Could you check a few things on this model? Use its own coordinates, in mm. A direction names the side the tool comes from. Coordinates: 2 decimals unless noted, no trailing zeros. Write each loop counter-clockwise with the first axis right and the second up, starting at its lowest first coordinate (ties: lowest second). Pieces come first, ordered by that corner, then holes. Notation, with made-up numbers: M -16,64 L 19,64 A21 cw 19,87 Z; hole C 37.5,-13 d11. An arc over 180 degrees is marked long. Write item = value, one per line.
```python
from build123d import *

# Parameters (mm, degrees)
SKETCH1_W                                            = 45
SKETCH1_H                                            = 48
BOSS_EXTRUDE1_DEPTH                                  = 6
SKETCH2_W                                            = 45
SKETCH2_H                                            = 15
BOSS_EXTRUDE2_DEPTH                                  = 10
CBORE_FOR_M3_HEXAGON_SOCKET_HEAD_CAP_SCR_D           = 3.4
CBORE_FOR_M3_HEXAGON_SOCKET_HEAD_CAP_SCR_DEPTH       = 15
CBORE_FOR_M3_HEXAGON_SOCKET_HEAD_CAP_SCR_CBORE_D     = 6
CBORE_FOR_M3_HEXAGON_SOCKET_HEAD_CAP_SCR_CBORE_DEPTH = 3.4
CBORE_FOR_M3_HEXAGON_SOCKET_HEAD_CAP_SCR_TIP         = 1.021463052
SKETCH6_W                                            = 5
SKETCH6_H                                            = 38
BOSS_EXTRUDE3_DEPTH                                  = 9
FILLET1_R                                            = 2
CBORE_FOR_M3_HEXAGON_SOCKET_HEAD_CAP_2_D             = 3.4
CBORE_FOR_M3_HEXAGON_SOCKET_HEAD_CAP_2_CBORE_D       = 6
CBORE_FOR_M3_HEXAGON_SOCKET_HEAD_CAP_2_CBORE_DEPTH   = 3.4
CHAMFER3_SIZE                                        = 3
CUT_EXTRUDE1_DEPTH                                   = 54.16013544
CUT_EXTRUDE1_DEPTH_BACK                              = 54.16013544
M3_TAPPED_HOLE1_D                                    = 2.5
M3_TAPPED_HOLE1_DEPTH                                = 4
M3_TAPPED_HOLE1_TIP                                  = 0.751075774


with BuildPart() as part:
    # Sketch1 → Boss-Extrude1 (new body)
    with BuildSketch(Plane.XY):
        Rectangle(SKETCH1_W, SKETCH1_H)
    extrude(amount=BOSS_EXTRUDE1_DEPTH)

    # Sketch2 → Boss-Extrude2 (add)
    with BuildSketch(Plane.XZ.offset(24)):
        with Locations((0, 7.5)):
            Rectangle(SKETCH2_W, SKETCH2_H)
    extrude(amount=-BOSS_EXTRUDE2_DEPTH)

    # CBORE for M3 Hexagon socket head cap scr
    with Locations(Plane(origin=(0, -14, 0), x_dir=(1, 0, 0), z_dir=(0, 1, 0))):
        with Locations((-11.5, -11.36), (11.5, -11.36)):
            CounterBoreHole(CBORE_FOR_M3_HEXAGON_SOCKET_HEAD_CAP_SCR_D / 2, CBORE_FOR_M3_HEXAGON_SOCKET_HEAD_CAP_SCR_CBORE_D / 2, CBORE_FOR_M3_HEXAGON_SOCKET_HEAD_CAP_SCR_CBORE_DEPTH, depth=CBORE_FOR_M3_HEXAGON_SOCKET_HEAD_CAP_SCR_DEPTH)
            with Locations((0, 0, -(CBORE_FOR_M3_HEXAGON_SOCKET_HEAD_CAP_SCR_DEPTH + CBORE_FOR_M3_HEXAGON_SOCKET_HEAD_CAP_SCR_TIP / 2))):  # 118° drill point
                Cone(0, CBORE_FOR_M3_HEXAGON_SOCKET_HEAD_CAP_SCR_D / 2, CBORE_FOR_M3_HEXAGON_SOCKET_HEAD_CAP_SCR_TIP, mode=Mode.SUBTRACT)

    # Sketch6 → Boss-Extrude3 (add)
    with BuildSketch(Plane.XY.offset(6)):
        with Locations((-20, 5)):
            Rectangle(SKETCH6_W, SKETCH6_H)
    extrude(amount=BOSS_EXTRUDE3_DEPTH)

    # Fillet1
    fillet1_edges = [part.edges().sort_by_distance(p)[0] for p in [
        (-17.5, -14, 10.5),
    ]]
    fillet(fillet1_edges, radius=FILLET1_R)

    # CBORE for M3 Hexagon socket head cap 2 (through all)
    with Locations(Plane.XY.offset(6)):
        with Locations((0, 19), (0, 4)):
            CounterBoreHole(CBORE_FOR_M3_HEXAGON_SOCKET_HEAD_CAP_2_D / 2, CBORE_FOR_M3_HEXAGON_SOCKET_HEAD_CAP_2_CBORE_D / 2, CBORE_FOR_M3_HEXAGON_SOCKET_HEAD_CAP_2_CBORE_DEPTH)

    # Chamfer3
    chamfer3_edges = [part.edges().sort_by_distance(p)[0] for p in [
        (22.5, -24, 7.5),
        (-22.5, -24, 7.5),
    ]]
    chamfer(chamfer3_edges, length=CHAMFER3_SIZE)

    # Sketch9 → Cut-Extrude1 (cut, two sides: drawn at the far end of the back side and taken through both)
    with BuildSketch(Plane(origin=(22.5, 0, 0), x_dir=(0, 0, -1), z_dir=(1, 0, 0)).offset(-CUT_EXTRUDE1_DEPTH_BACK)):
        Polygon((74.04249055, 101.04249055), (-3, 24), (-15, 12), (-92.04249055, -65.04249055), (-246.12747165, 89.04249055), (-80.04249055, 255.12747165), align=None)
    extrude(amount=CUT_EXTRUDE1_DEPTH + CUT_EXTRUDE1_DEPTH_BACK, mode=Mode.SUBTRACT)

    # M3 Tapped Hole1
    with Locations(Plane.XY.offset(6)):
        with Locations((-12.5, 16), (17.5, 16), (-12.5, -9), (17.5, -9)):
            Hole(M3_TAPPED_HOLE1_D / 2, depth=M3_TAPPED_HOLE1_DEPTH)
            with Locations((0, 0, -(M3_TAPPED_HOLE1_DEPTH + M3_TAPPED_HOLE1_TIP / 2))):  # 118° drill point
                Cone(0, M3_TAPPED_HOLE1_D / 2, M3_TAPPED_HOLE1_TIP, mode=Mode.SUBTRACT)


solid = part.part
```
Item 1: If we mould it in two halves opening along Z, with no side actions, what happens to faces 1 (the face through (0, 0, 0)), 2 (the face through (10.586, -20.746, 9.927)), 3 (the face through (-12.3, -9.08, 1.38)), 4 (the face through (-12.414, -20.746, 9.927))? For each: pulls with the +Z half, pulls with the -Z half, needs draft (parallel to the pull), parting line crosses it, or undercut.
Numbers:
face_1 = pulls with the -Z half
face_2 = undercut
face_3 = pulls with the +Z half
face_4 = undercut
Item 2: Imagine slicing it at C-C (x = 0). Write out the boundary of the cut face in (y, z), and give its area (3 significant figures).
Numbers:
outline = M -24,0 L 2.3,0 L 2.3,2.6 L 1,2.6 L 1,6 L -14,6 L -14,15 L -24,15 Z; M 5.7,0 L 17.3,0 L 17.3,2.6 L 16,2.6 L 16,6 L 7,6 L 7,2.6 L 5.7,2.6 Z; M 20.7,0 L 24,0 L 24,3 L 22,5 L 22,2.6 L 20.7,2.6 Z
area = 316 mm²
Item 3: Imagine slicing it at A-A (x = 11.5). Write out the boundary of the cut face in (y, z), and give its area (3 significant figures).
Numbers:
outline = M -24,0 L 24,0 L 24,3 L 21,6 L -14,6 L -14,8.36 L -17.4,8.36 L -17.4,9.66 L -24,9.66 Z; M -24,13.06 L -17.4,13.06 L -17.4,14.36 L -14,14.36 L -14,15 L -24,15 Z
area = 331 mm²
Item 4: Imagine slicing it at B-B (z = 11.36). Write out the boundary of the cut face in (x, y).
Numbers:
outline = M -22.5,-21 L -19.5,-24 L -13.2,-24 L -13.2,-17.4 L -14.5,-17.4 L -14.5,-14 L -15.5,-14 A2 cw -17.5,-12 L -17.5,15.64 L -22.5,15.64 Z; M -9.8,-24 L 9.8,-24 L 9.8,-17.4 L 8.5,-17.4 L 8.5,-14 L -8.5,-14 L -8.5,-17.4 L -9.8,-17.4 Z; M 13.2,-24 L 19.5,-24 L 22.5,-21 L 22.5,-14 L 14.5,-14 L 14.5,-17.4 L 13.2,-17.4 Z
Item 5: Imagine slicing it at D-D (y = -20). Write out the boundary of the cut face in (x, z).
Numbers:
outline = M -22.5,0 L 22.5,0 L 22.5,15 L -22.5,15 Z; hole C -11.5,11.36 d3.4; hole C 11.5,11.36 d3.4
Item 6: For faces 5 (the face through (2, 4, 2.6)), 6 (the face through (9.29, -15.68, 9.33)), 7 (the face through (-16.93, -13.4, 10.56)), which set-ups out of +Z, -Z, +X, -X, +Y, -Y let a thin tool reach every point of the face, with its end or its side?
Numbers:
face_5 = +Z
face_6 = +Y
face_7 = +Z, +X, +Y
Item 7: I'm going to push flat-ended pins straight in: P1, Ø5, axis at x = 18, y = -6, coming from the +Z side; P2, Ø4.5, axis at x = 11.5, z = 11.36, coming from the +Y side; P3, Ø3, axis at y = 0.5, z = 12.5, coming from the +X side. Where does each tip first touch, or does it pass through?
Numbers:
P1 = 6
P2 = -17.4
P3 = -17.5
Item 8: If I drill on line 1 along Y through (x, z) = (0, 0.7); line 2 along X through (y, z) = (-9, 4.8); line 3 along X through (y, z) = (-14.65, 11.36), over which ranges is the centre line in solid material (lowest first)?
Numbers:
line_1 = -24 to 2.3, 5.7 to 17.3, 20.7 to 24
line_2 = -22.5 to -13.75, -11.25 to 16.25, 18.75 to 22.5
line_3 = -22.5 to -14.5, -8.5 to 8.5, 14.5 to 22.5
